Job drawing, mm, ordinate dimensions from the low corner. One solid piece. A direction names the side the tool comes from. Coordinates: 2 decimals unless noted, no trailing zeros. Write each loop counter-clockwise with the first axis right and the second up, starting at its lowest first coordinate (ties: lowest second). Pieces come first, ordered by that corner, then holes.
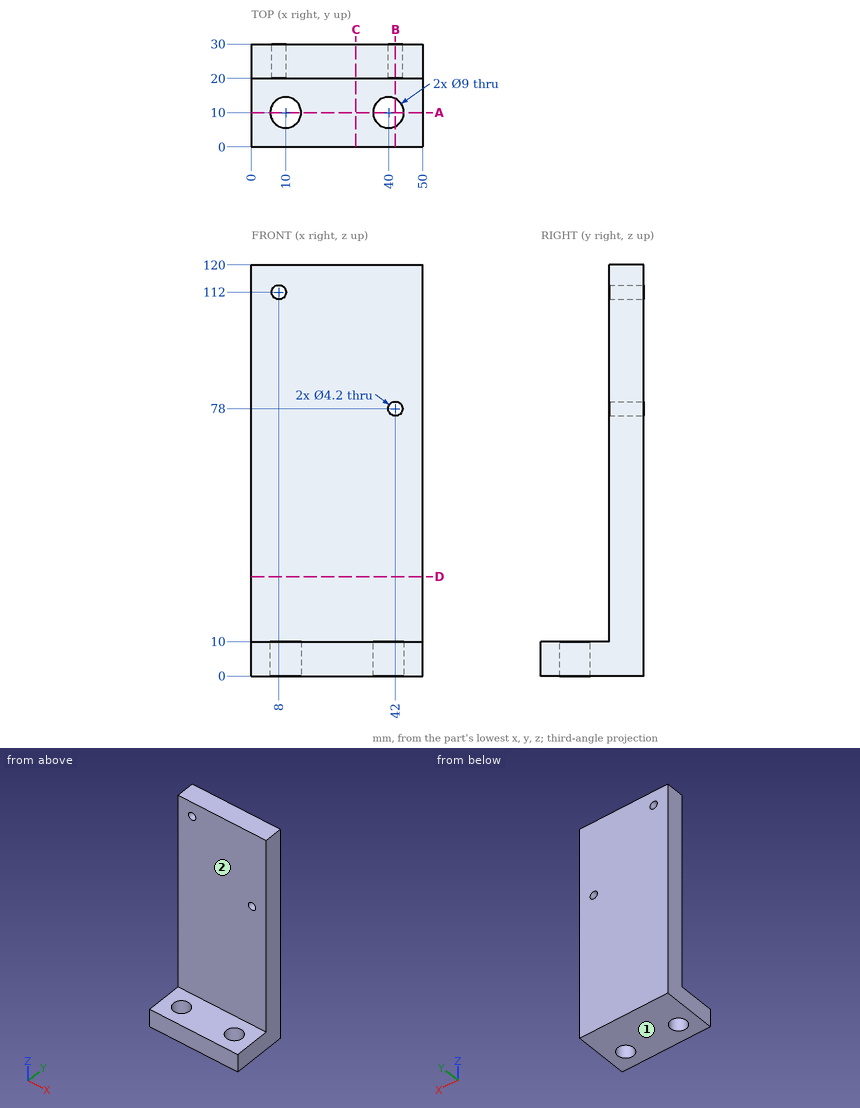
1. Saw through at A-A on y = 10. List the corners of the cut face in (x, z).
Computed values:
outline: (0, 0) - (5.5, 0) - (5.5, 10) - (0, 10) - close; (14.5, 0) - (35.5, 0) - (35.5, 10) - (14.5, 10) - close; (44.5, 0) - (50, 0) - (50, 10) - (44.5, 10) - close
2. Saw through at C-C on x = 30.5. List the corners of the cut face in (y, z), plus the area to 3 significant figures.
Computed values:
outline: (0, 0) - (30, 0) - (30, 120) - (20, 120) - (20, 10) - (0, 10) - close
area: 1,400 mm2
3. Saw through at B-B on x = 42. List the corners of the cut face in (y, z).
Computed values:
outline: (0, 0) - (5.97, 0) - (5.97, 10) - (0, 10) - close; (14.03, 0) - (30, 0) - (30, 75.9) - (20, 75.9) - (20, 10) - (14.03, 10) - close; (20, 80.1) - (30, 80.1) - (30, 120) - (20, 120) - close
4. Probe line 1 along Z through (x, y) = (42, 27.5); line 2 along Z through (x, y) = (8, 27.5); line 3 along Z through (x, y) = (36, 16.5). List the from-to ranges inside material, lowest first.
Computed values:
line 1: z = 0 to 75.9, 80.1 to 120
line 2: z = 0 to 109.9, 114.1 to 120
line 3: z = 0 to 10
5. 3-axis set-ups, long thin cutter, end or side, ignore diameter. For the marked faces 1 and 2: which of +Z, -Z, +X, -X, +Y, -Y reach the whole face in a straight line?
Computed values:
face 1: -Z, +X, -X, +Y, -Y
face 2: +Z, +X, -X, -Y
6. Saw through at D-D on z = 29. List the corners of the cut face in (x, y), plus the area to 3 significant figures.
Computed values:
outline: (0, 20) - (50, 20) - (50, 30) - (0, 30) - close
area: 500 mm2
7. Flat gauge pins, fed straight in: pin 1 (12 mm diameter, centred on x = 19, z = 87.5, fed in from -Y); pin 2 (1.5 mm diameter, centred on x = 6, y = 10, fed in from +Z). Where does each tip first touch, or does it go through?
Computed values:
pin 1: stops at y = 20
pin 2: stops at z = 10
